Autodesk Inventor part; units mm, degrees
ref_plane "YZ Plane" through (0, 0, 0) normal (1, 0, 0) x (0, 1, 0)
ref_plane "XZ Plane" through (0, 0, 0) normal (0, 1, 0) x (-1, 0, 0)
ref_plane "XY Plane" through (0, 0, 0) normal (0, 0, 1) x (1, 0, 0)
sketch "Skizze1" plane through (0, 0, 0) normal (0, 1, 0) x (-1, 0, 0)
  line L0 (63.5, -38) -> (-63.5, -38)
  line L1 (-63.5, -38) -> (-63.5, 38)
  line L2 (-63.5, 38) -> (63.5, 38)
  line L3 (63.5, 38) -> (63.5, -38)
  point P0 (0, 0)
  point P1 (0, -38)
  point P2 (63.5, 0)
  dimension "d0" = 76
  dimension "d1" = 127
extrude "Extrusion1" add sketch "Skizze1" along normal blind 2
sketch "Skizze2" plane through (0, 2, 0) normal (0, 1, 0) x (1, 0, 0)
  circle A0 centre (-58, 32.5) radius 2
  circle A1 centre (-58, -32.5) radius 2
  circle A2 centre (58, -32.5) radius 2
  circle A3 centre (58, 32.5) radius 2
  point P0 (0, 0)
  dimension "d4" = 4
  dimension "d5" = 4
  dimension "d6" = 4
  dimension "d7" = 4
  dimension "d8" = 116
  dimension "d9" = 58
  dimension "d10" = 65
  dimension "d11" = 32.5
extrude "Extrusion2" cut sketch "Skizze2" against normal through all
sketch "Skizze4" plane through (0, 2, 0) normal (0, 1, 0) x (1, 0, 0)
  line L0 (-54.6834, 37.5) -> (54.6834, 37.5)
  line L1 (63, 29.1834) -> (63, -29.1834)
  line L2 (54.6834, -37.5) -> (-54.6834, -37.5)
  line L3 (-63, -29.1834) -> (-63, 29.1834)
  line L4 (63.5, -38) -> (63.5, 38)
  line L5 (63.5, 38) -> (-63.5, 38)
  line L6 (-63.5, -38) -> (63.5, -38)
  line L7 (-63.5, 38) -> (-63.5, -38)
  circle A0 centre (-58, 32.5) radius 2
  circle A1 centre (-58, -32.5) radius 2
  arc A2 (-54.6834, -37.5) -> (-63, -29.1834) centre (-58, -32.5) ccw
  circle A3 centre (58, -32.5) radius 2
  arc A4 (63, -29.1834) -> (54.6834, -37.5) centre (58, -32.5) ccw
  arc A5 (54.6834, 37.5) -> (63, 29.1834) centre (58, 32.5) ccw
  circle A6 centre (58, 32.5) radius 2
  arc A7 (-63, 29.1834) -> (-54.6834, 37.5) centre (-58, 32.5) ccw
  point P0 (0, 0)
  point P1 (60.3979, -38)
  point P2 (63.5, -34.8979)
  point P3 (-60.3979, -38)
  dimension "d14" = 0.5
  dimension "d15" = 0.5
  dimension "d16" = 0.5
  dimension "d17" = 0.5
  dimension "d19" = 6
  dimension "d21" = 6
  dimension "d22" = 6
  dimension "d27" = 6
extrude "Extrusion3" add sketch "Skizze4" along normal blind 37 and the other way blind 4 contours L0 A5 L1 A4 L2 A2 L3 A7
equation "\"d5\" = d4"
equation "\"d6\" = d4"
equation "\"d7\" = d4"
equation "\"d14\" = d15"
equation "\"d16\" = d15"
equation "\"d17\" = d15"
equation "\"d19\" = d20"
equation "\"d21\" = d20"
equation "\"d22\" = d27"
properties part number "netzteil_12V"
Source: CAD feature listing. Evaluate the final solid. Frame: model axes, mm. A direction names the side the tool comes from. Round coordinates to 2 decimals unless told otherwise and drop trailing zeros. Order: outer loops, then holes, each group sorted by start corner. A loop starts at its lowest first (then second) coordinate and runs counter-clockwise, first axis right, second up. Notation, with made-up numbers: (-9.5, 71) -> (6.5, 71) arc R27 cw to (6.5, 90) -> close; hole circle Ø5 at (57.25, 31). An arc over 180 degrees is marked (long way). Use CSV: the item, a comma, the result in double quotes.
(1) Section C-C on y = 9. Return the cut outline in (x, z).
Report:
outline,"(-63, -29.18) arc R6 cw (long way) to (-54.68, -37.5) -> (54.68, -37.5) arc R6 cw (long way) to (63, -29.18) -> (63, 29.18) arc R6 cw (long way) to (54.68, 37.5) -> (-54.68, 37.5) arc R6 cw (long way) to (-63, 29.18) -> close"
(2) Section A-A on x = 58. Return the cut outline in (y, z), and give its area (3 significant figures).
Report:
outline,"(-2, -26.5) -> (0, -26.5) -> (0, -30.5) -> (2, -30.5) -> (2, -26.5) -> (39, -26.5) -> (39, 26.5) -> (2, 26.5) -> (2, 30.5) -> (0, 30.5) -> (0, 26.5) -> (-2, 26.5) -> close; (0, -38) -> (2, -38) -> (2, -34.5) -> (0, -34.5) -> close; (0, 34.5) -> (2, 34.5) -> (2, 38) -> (0, 38) -> close"
area,"2,200 mm^2"
(3) Section B-B on z = 32.5. Return the cut outline in (x, y).
Report:
outline,"(-63.5, 0) -> (-60, 0) -> (-60, 2) -> (-63.5, 2) -> close; (-56, 0) -> (-52, 0) -> (-52, -2) -> (52, -2) -> (52, 0) -> (56, 0) -> (56, 2) -> (52, 2) -> (52, 39) -> (-52, 39) -> (-52, 2) -> (-56, 2) -> close; (60, 0) -> (63.5, 0) -> (63.5, 2) -> (60, 2) -> close"
(4) Ray query, L1, parallel to Z at x = 58, y = 1.55; L2, parallel to Z at x = 58, y = -0.6; L3, parallel to X at y = 32, z = 32. Return the intervals inside material, ascending.
Report:
L1,"-38 to -34.5, -30.5 to 30.5, 34.5 to 38"
L2,"-26.5 to 26.5"
L3,"-52.02 to 52.02"
(5) First-contact query: pin 1 Ø5 at (x, z) = (-58, 32.5) entering from -Y; pin 2 Ø9.5 at (x, z) = (-58, -32.5) entering from +Y; pin 3 Ø10 at (x, y) = (-28, 22.5) entering from +Z; pin 4 Ø14 at (x, z) = (-58, 32.5) entering from -Y. Flat tips, straight axial feed; report the tip coordinate or a pass-through.
Report:
pin 1,"y = 0"
pin 2,"y = 2"
pin 3,"z = 37.5"
pin 4,"y = -2"
(6) Pull-direction query (Z, two-part tool) for faces 1 (the face through (-1, 20, -37.5)), 2 (the face through (1, 20, 37.5)), 3 (the face through (-63, 20, 0)), 4 (the face through (-57.077, 1.014, -30.726)); classes: +Z half, -Z half, draft (parallel to the pull), parting line (faces both ways), or undercut.
Report:
face 1,"-Z half"
face 2,"+Z half"
face 3,"draft"
face 4,"undercut"
(7) Access query for faces 5 (the face through (58.923, 1.014, 34.274)), 6 (the face through (53.864, -1.014, -28.154)), 7 (the face through (-53.654, 20.241, -28.364)), 8 (the face through (63, 20, 0)). Directions: +Z, -Z, +X, -X, +Y, -Y. A direction counts if a zero-diameter tool reaches every point of the face in a straight line with its end or side. Return the directions, or none.
Report:
face 5,"+Y, -Y"
face 6,"-Y"
face 7,"+Y"
face 8,"+Z, -Z, +X, +Y"
